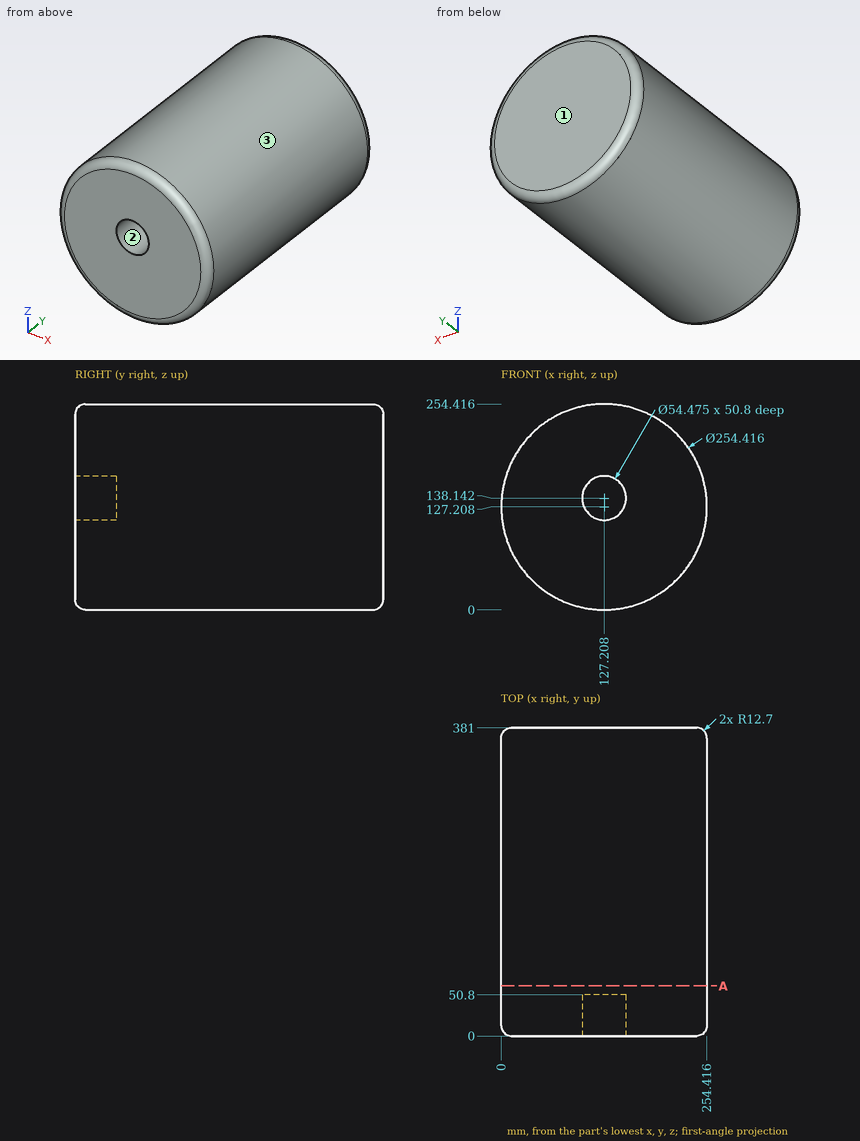
Print and shaded views of the part. All mm, measured from the part's lowest x, y and z. Coordinates: 2 decimals unless noted, no trailing zeros. Order: outer loops, then holes, each group sorted by start corner. A loop starts at its lowest first (then second) coordinate and runs counter-clockwise, first axis right, second up. Notation, with made-up numbers: (-33, 34) - (4, 34) arc R5 cw to (4, 43) - close; hole circle Ø4 at (34.25, -29.75). An arc over 180 degrees is marked (long way). Return JSON: item names as keys, results as strings. Group by question number.
Item 1: Drill centre lines: probe 1 along X at (y, z) = (222, 131.5); probe 2 along Z at (x, y) = (49.5, 287.5) (1 decimal); probe 3 along X at (y, z) = (77, 227.5) (1 decimal). Where is each one in solid material? Low to high. Write a range as from..to.
Item 2: Pin check, flat tips, straight feed: pin 1 (2 mm diameter, centred on x = 149, y = 72.5, fed in from -Z); pin 2 (4 mm diameter, centred on x = 165.5, y = 322.5, fed in from -Z); pin 3 (1.5 mm diameter, centred on y = 217, z = 63.5, fed in from -X). Stop position of each tip, or through.
Item 3: Cut at A-A (y = 62). List the corners of the cut face in (x, z).
Item 4: Pull direction X, two halves, no side cores. Call the marked faces 1, 2 and 3: pulls with the +X half, pulls with the -X half, needs draft (parallel to the pull), parting line crosses it, or undercut.
Check values:
{
 "1": {"probe 1": "x = 0.07..254.34", "probe 2": "z = 26.5..227.9", "probe 3": "x = 49..205.5"},
 "2": {"pin 1": "stops at z = 1.71", "pin 2": "stops at z = 5.29", "pin 3": "stops at x = 16.67"},
 "3": {"outline": "circle Ø254.42 at (127.21, 127.21)"},
 "4": {"face 1": "needs draft", "face 2": "undercut", "face 3": "parting line crosses it"}
}
